from build123d import *

# Parameters (mm, degrees)
F0_R     = 5
F1_DEPTH = 10.8
F2_R     = 5
F3_R     = 2.65
F4_DEPTH = 9


with BuildPart() as f1:
    # F0 (on Top) → F1 (new body)
    with BuildSketch(Plane.XY):
        Circle(F0_R)
    extrude(amount=F1_DEPTH)

    # F2
    f2_edges = [f1.edges().sort_by_distance(p)[0] for p in [
        (-5, 0, 10.8),
    ]]
    fillet(f2_edges, radius=F2_R)

    # F3 (on face) → F4 (cut)
    with BuildSketch(Plane(origin=(0, 0, 0), x_dir=(1, 0, 0), z_dir=(0, 0, -1))):
        Circle(F3_R)
    extrude(amount=-F4_DEPTH, mode=Mode.SUBTRACT)


solid = f1.part
Work out the finished part from the listing and answer in its coordinate system (mm). Round coordinates to 2 decimals unless told otherwise and drop trailing zeros. Write each loop counter-clockwise with the first axis right and the second up, starting at its lowest first coordinate (ties: lowest second). Pieces come first, ordered by that corner, then holes. Notation, with made-up numbers: (65.25, -14.5) - (85.25, -14.5) arc R17 ccw to (85.25, -0.5) - close; hole circle Ø9 at (-1, 63.5). An arc over 180 degrees is marked (long way). Answer in a Markdown table with one row per item. Add a question column.
1. Given pin 1 (2.5 mm diameter, centred on x = 1, y = -0.5, fed in from -Z); pin 2 (1 mm diameter, centred on x = 3.5, y = -3, fed in from +Z); pin 3 (1 mm diameter, centred on x = 3, z = 8, fed in from +Y); pin 4 (2 mm diameter, centred on x = 0.5, y = -0.5, fed in from +Z), each flat-ended and moving along its own axis, determine where each tip first touches the part or whether it passes through.
2. A cutting plane is placed at D-D, the plane x = 3. Determine the outline of the cut face in (y, z), and give its area (3 significant figures).
3. The mould has two halves that part along Y. Classify faces 1 (the flat face through (0, 0, 9)), 2 (the cylindrical face through (2.45, 1.01, 4.44)), 3 (the cylindrical face through (-1.08, -4.88, 2.86)), 4 (the flat face through (2, -2, 0)): +Y half, -Y half, draft (parallel to the pull), parting line (faces both ways), or undercut.
4. A cutting plane is placed at A-A, the plane y = 0. Determine the outline of the cut face in (x, z).
5. A cutting plane is placed at C-C, the plane z = 4.75. Determine the outline of the cut face in (x, y), and give its area (3 significant figures).
6. Find the intervals of material crossed by line 1 along Y through (x, z) = (0, 4); line 2 along Y through (x, z) = (-1.75, 0.5); line 3 along X through (y, z) = (1, 7.5), in increasing order. Write a range as from..to.
Worked out:
| question | item | result |
|---|---|---|
| 1 | pin 1 | z = 9 |
| 1 | pin 2 | z = 8.65 |
| 1 | pin 3 | y = 3.82 |
| 1 | pin 4 | z = 10.8 |
| 2 | outline | (-4, 0) - (4, 0) - (4, 5.8) arc R4 ccw to (-4, 5.8) - close |
| 2 | area | 71.5 mm^2 |
| 3 | face 1 | undercut |
| 3 | face 2 | undercut |
| 3 | face 3 | parting line |
| 3 | face 4 | draft |
| 4 | outline | (-5, 0) - (-2.65, 0) - (-2.65, 9) - (2.65, 9) - (2.65, 0) - (5, 0) - (5, 5.8) arc R5 ccw to (-5, 5.8) - close |
| 5 | outline | circle Ø10 at (0, 0); hole circle Ø5.3 at (0, 0) |
| 5 | area | 56.5 mm^2 |
| 6 | line 1 | -5..-2.65, 2.65..5 |
| 6 | line 2 | -4.68..-1.99, 1.99..4.68 |
| 6 | line 3 | -4.59..-2.45, 2.45..4.59 |
